from build123d import *
from build123d import SkipClean  # not in build123d's __all__

# Parameters (mm, degrees)
F0_R     = 14.2875
F1_DEPTH = 3.175
F3_DEPTH = 13.716


# Not quite as in the source:
# - a feature names something its author has since deleted; it is built from what else it names


with BuildPart() as f1:
    # F0 (on Front) → F1 (new body)
    with BuildSketch(Plane.XZ):
        with BuildLine():
            Line((-96.2781986811, -42.8291897772), (-4.2862845567, -50.6188479195))
            ThreePointArc((-4.2862845567, -50.6188479195), (50.4406573252, 6.0315908845), (-16.1005722699, 48.1810291773))
            Line((-16.1005722699, 48.1810291773), (-103.6621285019, 18.9207334083))
            ThreePointArc((-103.6621285019, 18.9207334083), (-125.3487825032, -11.3685027389), (-103.3274855148, -41.4153206587))
            ThreePointArc((-103.3274855148, -41.4153206587), (-99.8429919119, -42.3224346764), (-96.2781986811, -42.8291897772))
        make_face()
        with BuildLine():
            Line((-102.655842735, 15.9094190847), (-15.0942865031, 45.1697148537))
            ThreePointArc((-15.0942865031, 45.1697148537), (47.2881162424, 5.6546164542), (-4.0183917719, -47.4551699245))
            Line((-4.0183917719, -47.4551699245), (-96.0103058963, -39.6655117822))
            ThreePointArc((-96.0103058963, -39.6655117822), (-121.9721405786, -14.5851797), (-102.655842735, 15.9094190847))
        make_face(mode=Mode.SUBTRACT)
        with BuildLine():
            ThreePointArc((-4.0183917719, -47.4551699245), (47.2881162424, 5.6546164542), (-15.0942865031, 45.1697148537))
            Line((-15.0942865031, 45.1697148537), (-102.655842735, 15.9094190847))
            ThreePointArc((-102.655842735, 15.9094190847), (-121.9721405786, -14.5851797), (-96.0103058963, -39.6655117822))
            Line((-96.0103058963, -39.6655117822), (-4.0183917719, -47.4551699245))
        make_face()
        with Locations((-93.5992708332, -11.1924098275)):
            Circle(F0_R, mode=Mode.SUBTRACT)
        Circle(F0_R, mode=Mode.SUBTRACT)
    extrude(amount=F1_DEPTH)

    # F2 (on face) → F3 (join)
    with BuildSketch(Plane(origin=(0, 0, 0), x_dir=(-1, 0, 0), z_dir=(0, 1, 0))):
        with BuildLine():
            ThreePointArc((96.2781986811, -42.8291897772), (125.1246816615, -14.9621541303), (103.6621285019, 18.9207334083))
            Line((103.6621285019, 18.9207334083), (16.1005722699, 48.1810291773))
            ThreePointArc((16.1005722699, 48.1810291773), (-50.4406573252, 6.0315908845), (4.2862845567, -50.6188479195))
            Line((4.2862845567, -50.6188479195), (96.2781986811, -42.8291897772))
        make_face()
        with BuildLine():
            Line((15.0942865031, 45.1697148537), (102.655842735, 15.9094190847))
            ThreePointArc((102.655842735, 15.9094190847), (121.9721405786, -14.5851797), (96.0103058963, -39.6655117822))
            Line((96.0103058963, -39.6655117822), (4.0183917719, -47.4551699245))
            ThreePointArc((4.0183917719, -47.4551699245), (-47.2881162424, 5.6546164542), (15.0942865031, 45.1697148537))
        make_face(mode=Mode.SUBTRACT)
    with SkipClean():  # cleaning this boolean's faces spoils the solid; the shape is the same uncleaned
        extrude(amount=F3_DEPTH)


solid = f1.part
Design review of the part built by this model. Coordinates are the model's own, in mm. A direction names the side the tool comes from. Round coordinates to 2 decimals unless told otherwise and drop trailing zeros. Write each loop counter-clockwise with the first axis right and the second up, starting at its lowest first coordinate (ties: lowest second). Pieces come first, ordered by that corner, then holes. Notation, with made-up numbers: (66, 19.25) - (80, 19.25) arc R15 ccw to (80, 25.25) - close; hole circle Ø3 at (80, 19.25). An arc over 180 degrees is marked (long way). Use a Markdown table: item, result. Add a question column.
1. We need section A-A (x = 0). State the section outline as (y, z) points (1 decimal).
2. Wall thickness on probe 1 along Z at (x, y) = (0, 4.5) (3 decimals); probe 2 along X at (y, z) = (-0.25, -12); probe 3 along Z at (x, y) = (0, -2.3): over which ranges is each line inside the solid? List them lowest first.
3. Clearance check with flat-ended pins moving along their axes: pin 1 (1 mm diameter, centred on x = 10, y = 3, fed in from +Z); pin 2 (6 mm diameter, centred on y = 9, z = -1.5, fed in from +X); pin 3 (3 mm diameter, centred on y = 7.5, z = -35.5, fed in from +X). State where each tip first meets the part, or that it passes through.
4. We need section B-B (y = 6.5). State the section outline as (x, z) points (3 decimals).
5. For faces 3 (the face through (-122.032, 6.762, -14.041)), 4 (the face through (-50, 13.716, 34)), list the 3-axis set-ups (+Z, -Z, +X, -X, +Y, -Y) from which the entire face can be reached by the end or side of a thin tool; tool diameter is ignored.
6. We need section D-D (z = 30.5). State the section outline as (x, y) points (3 decimals), then the cut area to 3 significant figures.
7. Mouldability with a two-part tool opening along X and no side actions: class faces 1 (the face through (-80.4, -1.57, -16.66)), 2 (the face through (-19, -3.175, 1)) as +X half, -X half, draft (parallel to the pull), parting line (faces both ways), or undercut.
8. We need section C-C (z = 0). State the section outline as (x, y) points (1 decimal).
Output:
| question | item | result |
|---|---|---|
| 1 | outline | (-3.2, -50.8) - (13.7, -50.8) - (13.7, -47.6) - (0, -47.6) - (0, -14.3) - (-3.2, -14.3) - close; (-3.2, 14.3) - (0, 14.3) - (0, 47.6) - (13.7, 47.6) - (13.7, 50.8) - (-3.2, 50.8) - close |
| 2 | probe 1 | z = -50.8 to -47.625, 47.625 to 50.8 |
| 2 | probe 2 | x = -125.34 to -107.86, -79.33 to -7.75, 7.75 to 49.36 |
| 2 | probe 3 | z = -50.8 to -14.29, 14.29 to 50.8 |
| 3 | pin 1 | stops at z = 49.9 |
| 3 | pin 2 | stops at x = 50.8 |
| 3 | pin 3 | stops at x = 37.74 |
| 4 | outline | (-103.662, 18.921) arc R31.75 ccw to (-96.278, -42.829) - (-4.286, -50.619) arc R50.8 ccw (long way) to (-16.101, 48.181) - close; hole (-102.656, 15.909) arc R28.575 ccw to (-96.01, -39.666) - (-4.018, -47.455) arc R47.625 ccw (long way) to (-15.094, 45.17) - close |
| 5 | face 3 | +Y |
| 5 | face 4 | +Z, -Z, +X, -X, +Y |
| 6 | outline | (-69.011, -3.175) - (40.625, -3.175) - (40.625, 13.716) - (36.577, 13.716) - (36.577, 0) - (-58.993, 0) - (-58.993, 13.716) - (-69.011, 13.716) - close |
| 6 | area | 541 mm2 |
| 7 | face 1 | undercut |
| 7 | face 2 | draft |
| 8 | outline | (-123.3, -3.2) - (-102.5, -3.2) - (-102.5, 0) - (-119.9, 0) - (-119.9, 13.7) - (-123.3, 13.7) - close; (-84.7, -3.2) - (-14.3, -3.2) - (-14.3, 0) - (-84.7, 0) - close; (14.3, -3.2) - (50.8, -3.2) - (50.8, 13.7) - (47.6, 13.7) - (47.6, 0) - (14.3, 0) - close |
